Autodesk Inventor part; units mm, degrees
ref_plane "YZ Plane" through (0, 0, 0) normal (1, 0, 0) x (0, 1, 0)
ref_plane "XZ Plane" through (0, 0, 0) normal (0, 1, 0) x (-1, 0, 0)
ref_plane "XY Plane" through (0, 0, 0) normal (0, 0, 1) x (1, 0, 0)
sketch "Sketch1" plane through (0, 0, 0) normal (0, 0, 1) x (1, 0, 0)
  line L0 (-130, 67.5) -> (-130, -67.5)
  line L1 (-130, -67.5) -> (-120, -67.5)
  line L2 (-120, -67.5) -> (-120, -70)
  line L3 (-120, -70) -> (120, -70)
  line L4 (120, -70) -> (120, -67.5)
  line L5 (120, -67.5) -> (130, -67.5)
  line L6 (130, -67.5) -> (130, 67.5)
  line L7 (130, 67.5) -> (120, 67.5)
  line L8 (120, 67.5) -> (120, 72.5)
  line L9 (120, 72.5) -> (-120, 72.5)
  line L10 (-120, 72.5) -> (-120, 67.5)
  line L11 (-130, 67.5) -> (-120, 67.5)
  point P0 (0, 0)
  point P1 (0, 72.5)
  point P2 (130, 0)
  point P3 (-130, 0)
  dimension "d0" = 5
  dimension "d1" = 240
  dimension "d2" = 10
  dimension "d3" = 10
  dimension "d4" = 2.5
  dimension "d5" = 135
extrude "Extrusion1" add sketch "Sketch1" along normal blind 5
sketch "Sketch2" plane through (0, 0, 5) normal (0, 0, 1) x (1, 0, 0)
  line L0 (-76.75, -35.75) -> (-5.25, -35.75) construction
  line L1 (-5.25, -35.75) -> (-5.25, 35.75) construction
  line L2 (-5.25, 35.75) -> (-76.75, 35.75) construction
  line L3 (-76.75, 35.75) -> (-76.75, -35.75) construction
  line L4 (-76.75, -35.75) -> (-5.25, 35.75) construction
  line L5 (-5.25, -35.75) -> (-76.75, 35.75) construction
  line L6 (5.25, -35.75) -> (76.75, -35.75) construction
  line L7 (76.75, -35.75) -> (76.75, 35.75) construction
  line L8 (76.75, 35.75) -> (5.25, 35.75) construction
  line L9 (5.25, 35.75) -> (5.25, -35.75) construction
  line L10 (5.25, -35.75) -> (76.75, 35.75) construction
  line L11 (76.75, -35.75) -> (5.25, 35.75) construction
  point P0 (0, 0)
  point P1 (-41, 0)
  point P2 (41, 0)
  point P3 (-41, 0)
  point P4 (41, 0)
  point P5 (76.75, 35.75)
  dimension "d8" = 71.5
  dimension "d9" = 71.5
  dimension "d10" = 71.5
  dimension "d11" = 82
  dimension "d12" = 41
hole "Hole1" at (-76.75, 35.75, 5) at (-5.25, 35.75, 5) at (-5.25, -35.75, 5) at (-76.75, -35.75, 5) at (5.25, 35.75, 5) at (76.75, 35.75, 5) at (76.75, -35.75, 5) at (5.25, -35.75, 5) direction (0, 0, -1) diameter 4.5 depth 8 tip angle 118 countersink diameter 9.4 countersink angle 90
sketch "Sketch4" plane through (0, 0, 5) normal (0, 0, 1) x (1, 0, 0)
  circle A0 centre (-76.75, 35.75) radius 2.25
  circle A1 centre (-5.25, 35.75) radius 2.25
  circle A2 centre (5.25, 35.75) radius 2.25
  circle A3 centre (76.75, 35.75) radius 2.25
  circle A4 centre (76.75, -35.75) radius 2.25
  circle A5 centre (5.25, -35.75) radius 2.25
  circle A6 centre (-5.25, -35.75) radius 2.25
  circle A7 centre (-76.75, -35.75) radius 2.25
  circle A8 centre (-5.25, -35.75) radius 2.25 construction
  line L0 (-76.75, 35.75) -> (-5.25, 35.75) construction
  line L1 (-5.25, 35.75) -> (-5.25, -35.75) construction
  line L2 (-5.25, -35.75) -> (-76.75, -35.75) construction
  line L3 (-76.75, -35.75) -> (-76.75, 35.75) construction
  line L4 (5.25, -35.75) -> (76.75, -35.75) construction
  line L5 (76.75, -35.75) -> (76.75, 35.75) construction
  line L6 (76.75, 35.75) -> (5.25, 35.75) construction
  line L7 (5.25, 35.75) -> (5.25, -35.75) construction
  line L8 (-71, 0) -> (-11, 0)
  line L9 (-71, -2.5) -> (-11, -2.5)
  line L10 (-11, 2.5) -> (-71, 2.5)
  arc A9 (-71, 2.5) -> (-71, -2.5) centre (-71, 0) ccw
  arc A10 (-11, -2.5) -> (-11, 2.5) centre (-11, 0) ccw
  line L11 (-130, 67.5) -> (-130, -67.5) construction
  arc A11 (-11, -12.5) -> (-11, -7.5) centre (-11, -10) ccw
  line L12 (-71, -10) -> (-11, -10)
  line L13 (-71, -12.5) -> (-11, -12.5)
  line L14 (-11, -7.5) -> (-71, -7.5)
  arc A12 (-71, -7.5) -> (-71, -12.5) centre (-71, -10) ccw
  arc A13 (-11, -22.5) -> (-11, -17.5) centre (-11, -20) ccw
  line L15 (-71, -20) -> (-11, -20)
  line L16 (-71, -22.5) -> (-11, -22.5)
  line L17 (-11, -17.5) -> (-71, -17.5)
  arc A14 (-71, -17.5) -> (-71, -22.5) centre (-71, -20) ccw
  line L18 (-71, 7.5) -> (-11, 7.5)
  line L19 (-71, 10) -> (-11, 10)
  line L20 (-11, 12.5) -> (-71, 12.5)
  arc A15 (-11, 7.5) -> (-11, 12.5) centre (-11, 10) ccw
  arc A16 (-71, 12.5) -> (-71, 7.5) centre (-71, 10) ccw
  line L21 (-71, 17.5) -> (-11, 17.5)
  line L22 (-71, 20) -> (-11, 20)
  line L23 (-11, 22.5) -> (-71, 22.5)
  arc A17 (-11, 17.5) -> (-11, 22.5) centre (-11, 20) ccw
  arc A18 (-71, 22.5) -> (-71, 17.5) centre (-71, 20) ccw
  line L24 (0, 82.6384) -> (0, -86.5576) construction
  line L25 (71, 0) -> (11, 0)
  line L26 (71, -2.5) -> (11, -2.5)
  line L27 (11, 2.5) -> (71, 2.5)
  arc A19 (71, -2.5) -> (71, 2.5) centre (71, 0) ccw
  arc A20 (11, 2.5) -> (11, -2.5) centre (11, 0) ccw
  arc A21 (11, -7.5) -> (11, -12.5) centre (11, -10) ccw
  line L28 (71, -10) -> (11, -10)
  line L29 (71, -12.5) -> (11, -12.5)
  line L30 (11, -7.5) -> (71, -7.5)
  arc A22 (71, -12.5) -> (71, -7.5) centre (71, -10) ccw
  arc A23 (11, -17.5) -> (11, -22.5) centre (11, -20) ccw
  line L31 (71, -20) -> (11, -20)
  line L32 (71, -22.5) -> (11, -22.5)
  line L33 (11, -17.5) -> (71, -17.5)
  arc A24 (71, -22.5) -> (71, -17.5) centre (71, -20) ccw
  line L34 (71, 7.5) -> (11, 7.5)
  line L35 (71, 10) -> (11, 10)
  line L36 (11, 12.5) -> (71, 12.5)
  arc A25 (11, 12.5) -> (11, 7.5) centre (11, 10) ccw
  arc A26 (71, 7.5) -> (71, 12.5) centre (71, 10) ccw
  line L37 (71, 17.5) -> (11, 17.5)
  line L38 (71, 20) -> (11, 20)
  line L39 (11, 22.5) -> (71, 22.5)
  arc A27 (11, 22.5) -> (11, 17.5) centre (11, 20) ccw
  arc A28 (71, 17.5) -> (71, 22.5) centre (71, 20) ccw
  point P0 (0, 0)
  point P1 (-41, 0)
  point P2 (-41, -10)
  point P3 (-41, -20)
  point P4 (-41, 10)
  point P5 (-41, 20)
  point P6 (41, 0)
  point P7 (41, -10)
  point P8 (41, -20)
  point P9 (41, 10)
  point P10 (41, 20)
  dimension "d21" = 30
  dimension "d22" = 5
  dimension "d23" = 35.75
  dimension "d26" = 10
  dimension "d33" = 10
  dimension "d38" = 35.75
extrude "Extrusion2" cut sketch "Sketch4" against normal blind 5 contours A9 L10 A10 L9 | L13 A12 L14 A11 | L16 A14 L17 A13 | A16 L20 A15 L18 | A18 L23 A17 L21 | L26 A20 L27 A19 | L30 A22 L29 A21 | L33 A24 L32 A23 | L34 A25 L36 A26 | L37 A27 L39 A28
sketch "Sketch5" plane through (0, 0, 5) normal (0, 0, 1) x (1, 0, 0)
  point P0 (0, 0)
  point P1 (0, 50)
  point P2 (0, 50)
  dimension "d42" = 50
hole "Hole2" at (0, 50, 5) direction (0, 0, -1) diameter 10 depth 8 tip angle 118
equation "\"d39\" = d22"
properties part number "SeitenOben" material "Polycarbonate, Clear"
Read the model definition and answer for the solid it produces. Units are mm, in the model's axes. A direction names the side the tool comes from. Give positions to 0.01 mm unless a question says otherwise; leave off trailing zeros. Write each loop counter-clockwise with the first axis right and the second up, starting at its lowest first coordinate (ties: lowest second). Pieces come first, ordered by that corner, then holes. Notation, with made-up numbers: M 36.25,-11 L 54.25,-11 A18 cw 54.25,2 Z; hole C 8,27 d11. An arc over 180 degrees is marked long. Put each result on its own line as item: value. Start each with the question number.
1. The part is cut by section B-B, the plane z = 1.75. Give the number of separate pieces and of enclosed holes in the cut face, and give its area (3 significant figures).
2. The part is cut by section A-A, the plane y = -10. Give the vertices of the cut face in (x, z).
3. Consider line 1 along Y through (x, z) = (76.75, 0.8); line 2 along Y through (x, z) = (16, 2.6); line 3 along X through (y, z) = (35.75, 1.95). Determine where each line is inside the solid, lowest interval first.
4. Each of these flat-tipped pins is pushed along its axis until it touches: pin 1 Ø5 at (x, y) = (5.25, -35.75) entering from +Z; pin 2 Ø1.2 at (y, z) = (-69.5, 3) entering from +X; pin 3 Ø6 at (x, y) = (-76.75, 35.75) entering from +Z. Where does it stop, or does it pass through?
5. For a pull along X with two mould halves and no side action, classify faces 4 (the flat face through (130, -1, 2)), 5 (the flat face through (-41, -2.5, 3)), 6 (the flat face through (2, 72.5, 2)) as released by +X, released by -X, zero draft, split by the parting line, or undercut.
6. Which of the six approach directions +Z, -Z, +X, -X, +Y, -Y give full straight-line access (tool end or side, diameter ignored) to faces 1 (the flat face through (-2, 2, 5)), 2 (the flat face through (125, -67.5, 2)), 3 (the cylindrical face through (73.5, -0.1, 2.5))?
Final values:
1. separate pieces: 1
1. enclosed holes: 19
1. area: 33,500 mm²
2. outline: M -130,0 L -73.5,0 L -73.5,5 L -130,5 Z; M -8.5,0 L 8.5,0 L 8.5,5 L -8.5,5 Z; M 73.5,0 L 130,0 L 130,5 L 73.5,5 Z
3. line 1: y = -70 to -38, -33.5 to 33.5, 38 to 72.5
3. line 2: y = -70 to -22.5, -17.5 to -12.5, -7.5 to -2.5, 2.5 to 7.5, 12.5 to 17.5, 22.5 to 72.5
3. line 3: x = -130 to -79, -74.5 to -7.5, -3 to 3, 7.5 to 74.5, 79 to 130
4. pin 1: stops at z = 2.8
4. pin 2: stops at x = 120
4. pin 3: stops at z = 3.3
5. face 4: released by +X
5. face 5: undercut
5. face 6: zero draft
6. face 1: +Z, +X, -X, +Y, -Y
6. face 2: +Z, -Z, +X, -Y
6. face 3: +Z, -Z
